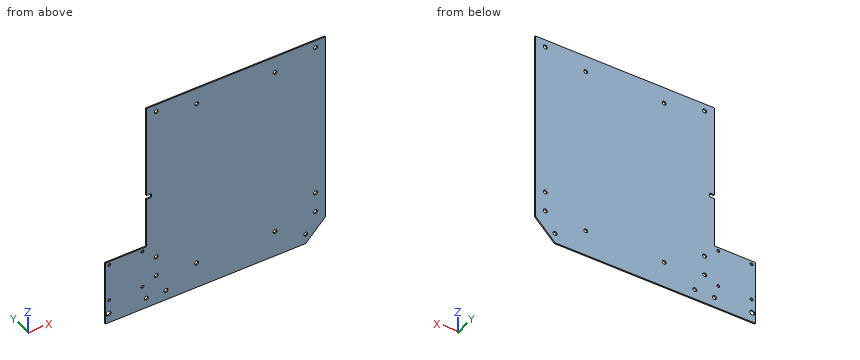
from build123d import *

# Parameters (mm, degrees)
BOSS_EXTRUDE1_DEPTH         = 1.5875
F_10_CLEARANCE_HOLE1_D      = 5.1054
F_1_4_0_25_DIAMETER_HOLE1_D = 6.35
F_6_CLEARANCE_HOLE1_D       = 3.6576
CUT_EXTRUDE1_DEPTH          = 306.201250484
F_10_CLEARANCE_HOLE2_D      = 4.9784


with BuildPart() as part:
    # Sketch3 → Boss-Extrude1 (new body)
    with BuildSketch(Plane(origin=(0, 0, 0), x_dir=(1, 0, 0), z_dir=(0, 1, 0))):
        with BuildLine():
            Line((-96.156504648, -3.621534833), (-96.156504648, 182.433465164))
            ThreePointArc((-96.156504648, 182.433465164), (-96.528479036, 183.331490776), (-97.426504648, 183.703465164))
            Line((-97.426504648, 183.703465164), (-149.179004653, 183.703465164))
            Line((-149.179004653, 183.703465164), (-149.179004653, 266.253465164))
            Line((-149.179004653, 266.253465164), (-70.756504695, 266.253465164))
            Line((-70.756504695, 266.253465164), (110.218495881, 266.253465164))
            Line((110.218495881, 266.253465164), (135.618495855, 240.853465164))
            Line((135.618495855, 240.853465164), (135.618495855, -3.621534833))
            Line((135.618495855, -3.621534833), (-96.156504648, -3.621534833))
        make_face()
    extrude(amount=BOSS_EXTRUDE1_DEPTH)

    # #10 Clearance Hole1 (through all)
    with Locations(Plane(origin=(0, 1.5875, 0), x_dir=(1, 0, 0), z_dir=(0, 1, 0))):
        with Locations((-83.456504653, -25.846534328), (-83.456504653, 202.75346618), (-83.456504653, 228.15346618), (-70.756504653, 253.55346618), (122.918495855, 202.753465164), (122.918495855, 228.153465164), (110.218495855, 253.553465164), (-83.456504653, 5.903465672), (122.918495855, 5.903465672), (-96.15650472, 253.553466178)):
            Hole(F_10_CLEARANCE_HOLE1_D / 2)

    # 1/4 (0.25) Diameter Hole1 (through all)
    with Locations(Plane(origin=(0, 0, 0), x_dir=(-1, 0, 0), z_dir=(0, -1, 0))):
        with Locations((145.369004653, 253.553465164)):
            Hole(F_1_4_0_25_DIAMETER_HOLE1_D / 2)

    # #6 Clearance Hole1 (through all)
    with Locations(Plane(origin=(0, 1.5875, 0), x_dir=(1, 0, 0), z_dir=(0, 1, 0))):
        with Locations((-144.305157527, 235.976041671), (-144.305157527, 188.226395138), (-101.258714708, 188.226395138), (-101.258714708, 235.978395138)):
            Hole(F_6_CLEARANCE_HOLE1_D / 2)

    # Sketch17 → Cut-Extrude1 (cut, through all)
    with BuildSketch(Plane(origin=(0, 1.5875, 0), x_dir=(1, 0, 0), z_dir=(0, 1, 0))):
        with BuildLine():
            Line((-96.156504648, 114.361465167), (-91.076504648, 114.361465167))
            ThreePointArc((-91.076504648, 114.361465167), (-90.178479036, 114.733439555), (-89.806504648, 115.631465167))
            Line((-89.806504648, 115.631465167), (-89.806504648, 118.171465167))
            ThreePointArc((-89.806504648, 118.171465167), (-90.178479036, 119.069490779), (-91.076504648, 119.441465167))
            Line((-91.076504648, 119.441465167), (-96.156504648, 119.441465167))
            Line((-96.156504648, 119.441465167), (-96.156504648, 114.361465167))
        make_face()
    extrude(amount=-CUT_EXTRUDE1_DEPTH, mode=Mode.SUBTRACT)

    # #10 Clearance Hole2 (through all)
    with Locations(Plane(origin=(0, 1.5875, 0), x_dir=(1, 0, 0), z_dir=(0, 1, 0))):
        with Locations((-31.069004399, 233.22189625), (70.530995601, 233.22189625), (70.530995601, 17.32189625), (-31.069004399, 17.32189625)):
            Hole(F_10_CLEARANCE_HOLE2_D / 2)


solid = part.part
CAD build for the part. Positions are in the model's coordinates, mm. Coordinates: 2 decimals unless noted, no trailing zeros. Write each loop counter-clockwise with the first axis right and the second up, starting at its lowest first coordinate (ties: lowest second). Pieces come first, ordered by that corner, then holes. Notation, with made-up numbers: (-16.75, 32) - (40.25, 32) arc R9 ccw to (40.25, 38) - close; hole circle Ø11 at (-18.5, 61). An arc over 180 degrees is marked (long way). Use a Markdown table: item, result. Add a question column.
Item 1: Band-saw the part on C-C, the plane x = -113. Give the cut face in (y, z), and give its area (3 significant figures).
Item 2: Band-saw the part on A-A, the plane y = 0.75. Give the number of separate pieces and of enclosed holes in the cut face, and give its area (3 significant figures).
Item 3: Drill centre lines: L1, parallel to X at y = 0.75, z = -155.5; L2, parallel to Z at x = -29, y = 0.7; L3, parallel to X at y = 0.4, z = -114.5. Where is each one in solid material? Low to high. Write a range as from..to.
Item 4: Flat gauge pins, fed straight in: pin 1 (0.8 mm diameter, centred on y = 1, z = -117, fed in from -X); pin 2 (0.8 mm diameter, centred on y = 1, z = -36.5, fed in from -X). Where does each tip first touch, or does it go through?
Item 5: Band-saw the part on B-B, the plane z = -136.5. Give the cut face in (x, y), and give its area (3 significant figures).
Numbers:
| question | item | result |
|---|---|---|
| 1 | outline | (0, -266.25) - (1.59, -266.25) - (1.59, -183.7) - (0, -183.7) - close |
| 1 | area | 131 mm2 |
| 2 | separate pieces | 1 |
| 2 | enclosed holes | 18 |
| 2 | area | 66,200 mm2 |
| 3 | L1 | -96.16..135.62 |
| 3 | L2 | -266.25..-234.61, -231.84..-18.71, -15.94..3.62 |
| 3 | L3 | -90.5..135.62 |
| 4 | pin 1 | x = -89.81 |
| 4 | pin 2 | x = -96.16 |
| 5 | outline | (-96.16, 0) - (135.62, 0) - (135.62, 1.59) - (-96.16, 1.59) - close |
| 5 | area | 368 mm2 |
